Job drawing, mm, ordinate dimensions from the low corner. One solid piece. A direction names the side the tool comes from. Give positions to 0.01 mm unless a question says otherwise; leave off trailing zeros. Loops run counter-clockwise (first coordinate to the right, second up) from the corner with the lowest first, then second, coordinate; pieces in that order, holes last. Notation, with made-up numbers: M 20.25,30.5 L 56.25,30.5 A6 ccw 56.25,40.5 Z; hole C 8,-17 d11. An arc over 180 degrees is marked long. One line per question, with ' | ' between items.
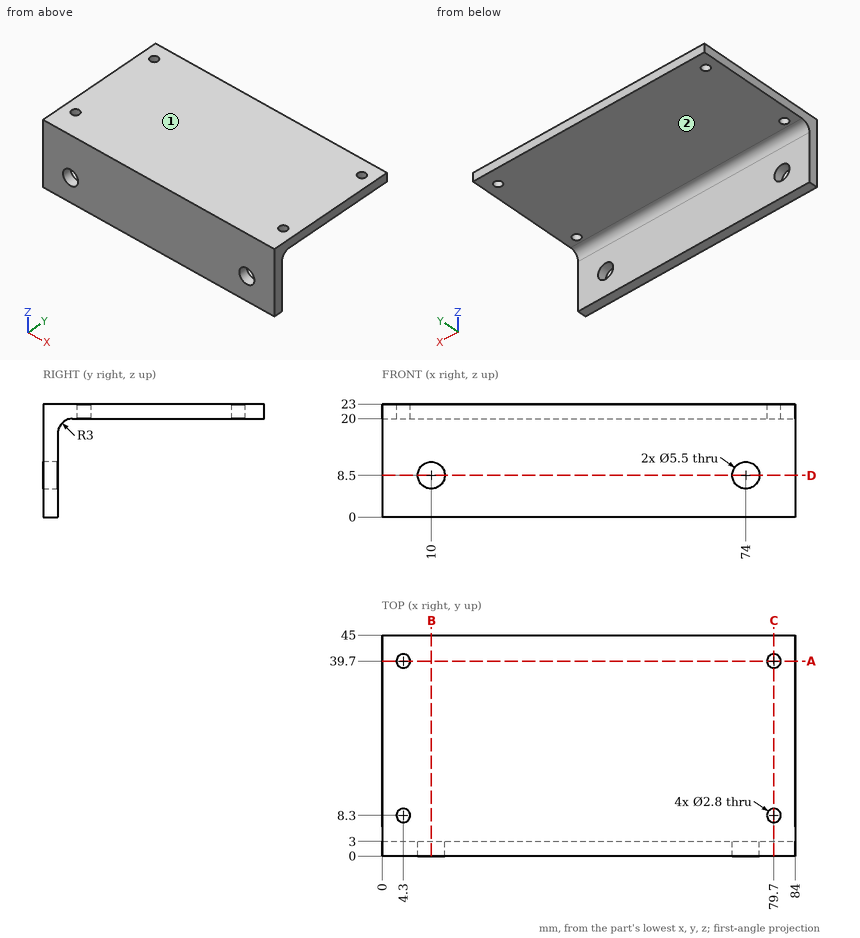
Item 1: Drill centre lines: line 1 along Y through (x, z) = (4.3, 22); line 2 along X through (y, z) = (1.4, 8.5); line 3 along Z through (x, y) = (74, 2). Where is each one in solid material? Low to high. Write a range as [from, to].
Conclusion:
line 1: [0, 6.9], [9.7, 38.3], [41.1, 45] | line 2: [0, 7.25], [12.75, 71.25], [76.75, 84] | line 3: [0, 5.75], [11.25, 23]
Item 2: Drop flat-ended pins along their axis: P1, Ø5, axis at x = 10, z = 8.5, coming from the +Y side; P2, Ø7, axis at x = 74, z = 8.5, coming from the +Y side; P3, Ø5, axis at y = 33.5, z = 19.5, coming from the +X side; P4, Ø4.5, axis at x = 4.3, y = 8.3, coming from the -Z side. Give the stop position or say it passes through.
Conclusion:
P1: through | P2: y = 3 | P3: x = 84 | P4: z = 20
Item 3: Saw through at D-D on z = 8.5. Give the cut face in (x, y).
Conclusion:
outline: M 0,0 L 7.25,0 L 7.25,3 L 0,3 Z; M 12.75,0 L 71.25,0 L 71.25,3 L 12.75,3 Z; M 76.75,0 L 84,0 L 84,3 L 76.75,3 Z
Item 4: Saw through at C-C on x = 79.7. Give the cut face in (y, z).
Conclusion:
outline: M 0,0 L 3,0 L 3,17 A3 cw 6,20 L 6.9,20 L 6.9,23 L 0,23 Z; M 9.7,20 L 38.3,20 L 38.3,23 L 9.7,23 Z; M 41.1,20 L 45,20 L 45,23 L 41.1,23 Z
Item 5: Saw through at B-B on x = 10. Give the cut face in (y, z), and give its area (3 significant figures).
Conclusion:
outline: M 0,0 L 3,0 L 3,5.75 L 0,5.75 Z; M 0,11.25 L 3,11.25 L 3,17 A3 cw 6,20 L 45,20 L 45,23 L 0,23 Z | area: 180 mm²
Item 6: 3-axis set-ups, long thin cutter, end or side, ignore diameter. For the marked faces 1 and 2: which of +Z, -Z, +X, -X, +Y, -Y reach the whole face in a straight line?
Conclusion:
face 1: +Z, +X, -X, +Y, -Y | face 2: -Z, +X, -X, +Y
Item 7: Saw through at A-A on y = 39.7. Give the cut face in (x, z).
Conclusion:
outline: M 0,20 L 2.9,20 L 2.9,23 L 0,23 Z; M 5.7,20 L 78.3,20 L 78.3,23 L 5.7,23 Z; M 81.1,20 L 84,20 L 84,23 L 81.1,23 Z
